The figure shows three views and two pictorial views of one solid part (mm, origin at its lowest corner). Answer the questions. Coordinates: 2 decimals unless noted, no trailing zeros. Write each loop counter-clockwise with the first axis right and the second up, starting at its lowest first coordinate (ties: lowest second). Pieces come first, ordered by that corner, then holes.
Item 1: Each of these flat-tipped pins is pushed along its axis until it touches: P1, Ø12, axis at y = 12.5, z = 28.5, coming from the +X side; P2, Ø12, axis at y = 13.5, z = 30, coming from the +X side. Where does it stop, or does it pass through?
Item 2: Straight lines are drawn through the part: probe 1 along Z at (x, y) = (429, 47); probe 2 along Z at (x, y) = (61, 20); probe 3 along X at (y, z) = (13, 17). For each, find the intervals that lie inside material, in ascending order.
Item 3: Section A-A (y = 13.5) is taken. Give the vertices of the cut face in (x, z).
Item 4: Section B-B (x = 423) is taken. Give the vertices of the cut face in (y, z).
Item 5: Section C-C (z = 23) is taken. Give the vertices of the cut face in (x, y).
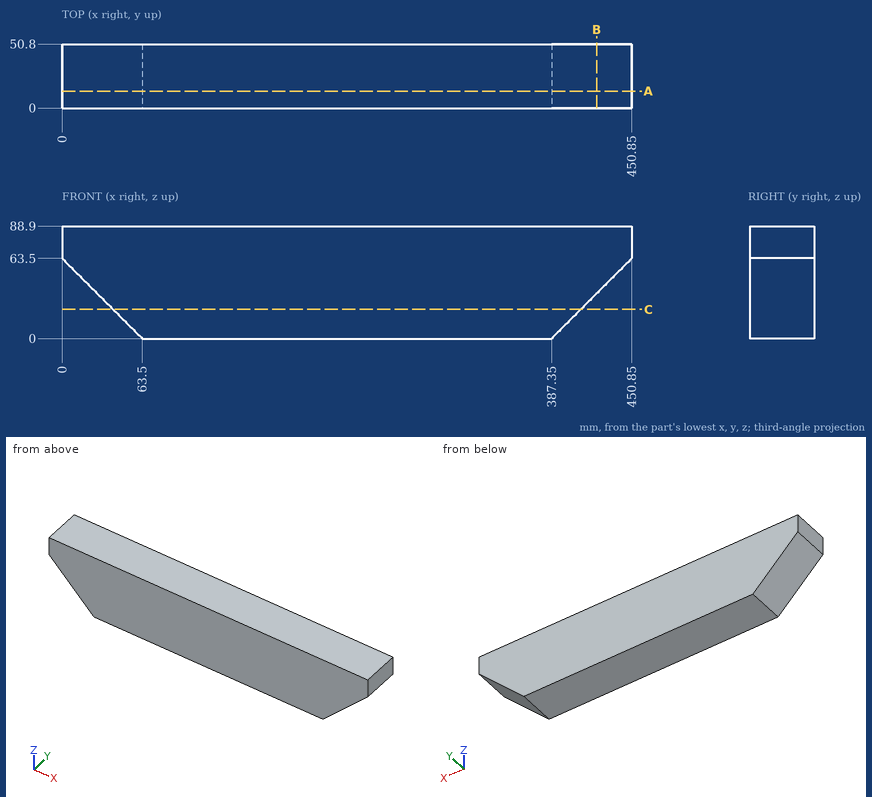
Established:
1. P1: stops at x = 421.85
1. P2: stops at x = 423.35
2. probe 1: z = 41.65 to 88.9
2. probe 2: z = 2.5 to 88.9
2. probe 3: x = 46.5 to 404.35
3. outline: (0, 63.5) - (63.5, 0) - (387.35, 0) - (450.85, 63.5) - (450.85, 88.9) - (0, 88.9) - close
4. outline: (0, 35.65) - (50.8, 35.65) - (50.8, 88.9) - (0, 88.9) - close
5. outline: (40.5, 0) - (410.35, 0) - (410.35, 50.8) - (40.5, 50.8) - close
